Design review of the part built by this model. Coordinates are the model's own, in mm. A direction names the side the tool comes from. Give positions to 0.01 mm unless a question says otherwise; leave off trailing zeros. Order: outer loops, then holes, each group sorted by start corner. A loop starts at its lowest first (then second) coordinate and runs counter-clockwise, first axis right, second up. Notation, with made-up numbers: M -2.75,10 L 28.25,10 A17 ccw 28.25,36 Z; hole C 25.25,38 d3. An arc over 180 degrees is marked long. Answer as a JSON object with one key per item and string values.
from build123d import *

# Parameters (mm, degrees)
F0_W     = 101.6
F0_H     = 50.8
F1_DEPTH = 127
F2_R     = 4.7625
F3_DEPTH = 158.242
F4_R     = 12.7
F5_SIZE  = 5.08


with BuildPart() as f1:
    # F0 (on Front) → F1 (new body)
    with BuildSketch(Plane.XZ):
        Rectangle(F0_W, F0_H)
    extrude(amount=F1_DEPTH)

    # F2 (on face) → F3 (cut)
    with BuildSketch(Plane(origin=(0, 0, 0), x_dir=(-1, 0, 0), z_dir=(0, 1, 0))):
        with Locations((31.891733, -12.221986)):
            Circle(F2_R)
        with Locations((11.267137, -12.221986)):
            Circle(F2_R)
    extrude(amount=-F3_DEPTH, mode=Mode.SUBTRACT)

    # F4
    f4_edges = [f1.edges().sort_by_distance(p)[0] for p in [
        (-50.8, -63.5, 25.4),
    ]]
    fillet(f4_edges, radius=F4_R)

    # F5
    f5_edges = [f1.edges().sort_by_distance(p)[0] for p in [
        (50.8, -63.5, 25.4),
        (-50.8, -63.5, -25.4),
    ]]
    chamfer(f5_edges, length=F5_SIZE)

    # F0 (on Front) → F6 (revolve)
    with BuildSketch(Plane.XZ):
        Rectangle(F0_W, F0_H)
    revolve(axis=Axis((0, 0, 25.4), (-1, 0, 0)))


solid = f1.part
(1) Draft analysis for pull direction Z (two halves, no side actions). For faces 4 (the flat face through (2, -63, -25.4)), 5 (the flat face through (50.8, -20, 15)), 6 (the flat face through (3, -88, 25.4)), 7 (the cylindrical face through (-31.8, -33.6, -12.7)), state which applies: +Z half, -Z half, draft (parallel to the pull), parting line (faces both ways), or undercut.
Checked values:
{"face 4": "-Z half", "face 5": "draft", "face 6": "+Z half", "face 7": "undercut"}
(2) We need section B-B (y = 18). Write out the cut boundary in (x, z), plus the area to 3 significant figures.
Checked values:
{"outline": "M -50.8,-22.1 L 50.8,-22.1 L 50.8,72.9 L -50.8,72.9 Z", "area": "9,650 mm^2"}
(3) To check wall thickness, follow L1, parallel to Z at x = 0.5, y = -80; L2, parallel to Y at x = -16, z = 63; L3, parallel to Z at x = -14.5, y = -67. State the ranges of each line that lie inside material, in increasing order. Write a range as from..to.
Checked values:
{"L1": "z = -25.4..25.4", "L2": "y = -34.16..34.16", "L3": "z = -25.4..-15.72, -8.72..25.4"}
(4) Tool access review of faces 1 (the flat face through (-48.22, -62.61, -22.9)), 2 (the flat face through (-50.8, -20, 15)), 3 (the cylindrical face through (-10.23, -76.81, -16.87)): name each direction out of +Z, -Z, +X, -X, +Y, -Y from which nothing blocks a thin tool from reaching the whole face with its end or side.
Checked values:
{"face 1": "-Z, -X, -Y", "face 2": "+Z, -Z, -X, +Y, -Y", "face 3": "-Y"}
(5) We need section A-A (x = 22.5). Write out the cut boundary in (y, z).
Checked values:
{"outline": "M -127,-25.4 L 0,-25.4 A50.8 ccw long -50.8,25.4 L -127,25.4 Z"}
(6) Insertion check: pin 1 (12 mm diameter, centred on x = -14.5, z = 65, fed in from +Y); pin 2 (10 mm diameter, centred on x = -39, y = 6, fed in from +Z); pin 3 (3 mm diameter, centred on x = 32.5, z = 8.5, fed in from +Y). Each pin has a flat end and moves straight along its axis. Give the tip position at first contact, or say it passes through.
Checked values:
{"pin 1": "stops at y = 38.1", "pin 2": "stops at z = 76.19", "pin 3": "stops at y = 48.41"}
